CAD build for the part. Positions are in the model's coordinates, mm. A direction names the side the tool comes from. Coordinates: 2 decimals unless noted, no trailing zeros. Write each loop counter-clockwise with the first axis right and the second up, starting at its lowest first coordinate (ties: lowest second). Pieces come first, ordered by that corner, then holes. Notation, with made-up numbers: M -4,14.5 L 10,14.5 A18 ccw 10,35.5 Z; hole C 15.5,65.5 d6. An arc over 180 degrees is marked long. Answer as CSV lines item,"result". Start each with the question number.
```python
from build123d import *

# Parameters (mm, degrees)
F2_R     = 7.270103
F3_DEPTH = 55.001


with BuildPart() as f1:
    # F0 (on Front) → F1 (revolve)
    with BuildSketch(Plane.XZ):
        with BuildLine():
            Line((14.738567, 48.729044), (0, 48.729044))
            Line((0, 48.729044), (0, -6.270956))
            Line((0, -6.270956), (25, -6.270956))
            ThreePointArc((25, -6.270956), (27.765735, -5.436374), (29.608177, -3.21124))
            Line((29.608177, -3.21124), (30.131203, -1.969053))
            ThreePointArc((30.131203, -1.969053), (30.522956, -0.002314), (30.110414, 1.96017))
            Line((30.110414, 1.96017), (26.946491, 9.257603))
            ThreePointArc((26.946491, 9.257603), (25.609479, 11.068015), (23.613915, 12.10865))
            Line((23.613915, 12.10865), (19.738567, 13.11337))
            Line((19.738567, 13.11337), (19.738567, 43.729044))
            ThreePointArc((19.738567, 43.729044), (18.274101, 47.264578), (14.738567, 48.729044))
        make_face()
    revolve(axis=Axis((0, 0, 21.229044), (0, 0, 1)))

    # F2 (on face) → F3 (cut, through all)
    with BuildSketch(Plane.XY.offset(48.729044)):
        Circle(F2_R)
    extrude(amount=-F3_DEPTH, mode=Mode.SUBTRACT)


solid = f1.part
```
1) Pin check, flat tips, straight feed: P1, Ø5, axis at x = -11, z = -0.5, coming from the +Y side; P2, Ø1.5, axis at x = -4, y = 4.5, coming from the -Z side; P3, Ø4, axis at y = -16.5, z = 23.5, coming from the -X side; P4, Ø10, axis at y = 13, z = 1, coming from the +X side. Stop position of each tip, or through.
2) Band-saw the part on A-A, the plane x = 0. List the corners of the cut face in (y, z), plus the area to 3 significant figures.
3) Band-saw the part on C-C, the plane z = 21.5. List the corners of the cut face in (x, y).
4) Two-plate mould, pull along X, no slides. Class faces 1 (the cylindrical face through (-1.576, -7.097, 21.614)), 2 (the flat face through (-7, -3, 48.729)), 3 (the conical face through (-21.5, -16.5, 8.9)): pulls with the +X half, pulls with the -X half, needs draft (parallel to the pull), parting line crosses it, or undercut.
5) Tool access for faces 4 (the cylindrical face through (18.827, 5.929, 28.636)), 5 (the flat face through (-5, 6, -6.271)): list every direction of +Z, -Z, +X, -X, +Y, -Y with a clear straight run to the whole face (end or side of a thin tool).
6) Probe L1, parallel to Y at x = 0, z = 24.5; L2, parallel to Y at x = 0, z = 6; L3, parallel to X at y = 2.5, z = 40.5. List the from-to ranges inside material, lowest first. Write a range as [from, to].
Result sheet:
1,P1,"stops at y = 29.31"
1,P2,"passes through"
1,P3,"stops at x = -13.39"
1,P4,"stops at x = 29.43"
2,outline,"M -30.13,-1.97 L -29.61,-3.21 A5 ccw -25,-6.27 L -7.27,-6.27 L -7.27,48.73 L -14.74,48.73 A5 ccw -19.74,43.73 L -19.74,13.11 L -23.61,12.11 A5 ccw -26.95,9.26 L -30.11,1.96 A5 ccw Z; M 7.27,-6.27 L 25,-6.27 A5 ccw 29.61,-3.21 L 30.13,-1.97 A5 ccw 30.11,1.96 L 26.95,9.26 A5 ccw 23.61,12.11 L 19.74,13.11 L 19.74,43.73 A5 ccw 14.74,48.73 L 7.27,48.73 Z"
2,area,"1,690 mm²"
3,outline,"C 0,0 d39.48; hole C 0,0 d14.54"
4,face 1,"undercut"
4,face 2,"needs draft"
4,face 3,"parting line crosses it"
5,face 4,"+Z"
5,face 5,"-Z, +X, -X, +Y, -Y"
6,L1,"y = [-19.74, -7.27], [7.27, 19.74]"
6,L2,"y = [-28.36, -7.27], [7.27, 28.36]"
6,L3,"x = [-19.58, -6.83], [6.83, 19.58]"
